Here's how the part is built. I have some questions about the finished solid (model axes, mm). A direction names the side the tool comes from. Give positions to 0.01 mm unless a question says otherwise; leave off trailing zeros. Write each loop counter-clockwise with the first axis right and the second up, starting at its lowest first coordinate (ties: lowest second). Pieces come first, ordered by that corner, then holes. Notation, with made-up numbers: (57.5, 82) -> (72.5, 82) arc R22 cw to (72.5, 120) -> close; hole circle Ø10 at (16.5, 12). An arc over 180 degrees is marked (long way). Return JSON: item names as keys, results as strings.
from build123d import *

# Parameters (mm, degrees)
BOSS_EXTRUDE5_DEPTH = 19
BOSS_EXTRUDE6_DEPTH = 8
BOSS_EXTRUDE7_DEPTH = 6.325904881
SKETCH11_R          = 1.75
CUT_MOTOR_DEPTH     = 19
SKETCH12_R          = 1.5
CUT_EXTRUDE7_DEPTH  = 46.325937613
SKETCH13_R          = 2.25
CUT_EXTRUDE8_DEPTH  = 46.216453805
SKETCH14_R          = 5.5
CUT_EXTRUDE9_DEPTH  = 4
SKETCH16_R          = 11.5
CUT_MOTOR_L_DEPTH   = 2.5
CUT_MOTOR_R_START   = -2.5
SKETCH15_R          = 11.5
CUT_MOTOR_R_DEPTH   = 2.5
SKETCH19_R          = 3.25
CUT_EXTRUDE10_DEPTH = 8
SKETCH20_R          = 2.75
CUT_EXTRUDE11_DEPTH = 62.878766896
CUT_EXTRUDE12_DEPTH = 56.924303306
FILLET1_R           = 2
FILLET2_R           = 1.5
FILLET3_R           = 1.5
SKETCH24_R          = 1.75
CUT_EXTRUDE14_DEPTH = 6
CUT_EXTRUDE15_DEPTH = 2.5


with BuildPart() as part:
    # Sketch10 → Boss-Extrude5 (new, symmetric)
    with BuildSketch(Plane(origin=(0, 0, 0), x_dir=(0, 0, -1), z_dir=(1, 0, 0))):
        with BuildLine():
            Line((-27.445904881, 9.607875665), (-20.588029216, 9.607875665))
            Line((-20.588029216, 9.607875665), (-17.838029216, 6.857875665))
            Line((-17.838029216, 6.857875665), (-17.838029216, 0))
            Line((-17.838029216, 0), (0.18, 0))
            Line((0.18, 0), (0.18, -25))
            Line((0.18, -25), (6.18, -25))
            Line((6.18, -25), (6.18, -6.648603252))
            Line((6.18, -6.648603252), (9.067622319, -3.148603252))
            Line((9.067622319, -3.148603252), (13.795773677, -3.148603252))
            ThreePointArc((13.795773677, -3.148603252), (19.7879876, -3.62453907), (22.93, 1.5))
            Line((22.93, 1.5), (22.93, 17.5))
            Line((22.93, 17.5), (-21.12, 17.5))
            Line((-21.12, 17.5), (-21.12, 25.5))
            Line((-21.12, 25.5), (-27.445904881, 25.5))
            Line((-27.445904881, 25.5), (-27.445904881, 9.607875665))
        make_face()
    extrude(amount=BOSS_EXTRUDE5_DEPTH, both=True)

    # Sketch18 → Boss-Extrude6 (add)
    with BuildSketch(Plane(origin=(0, 17.5, 0), x_dir=(1, 0, 0), z_dir=(0, 1, 0))):
        Polygon((-3.75, 22.93), (3.75, 22.93), (3.75, -21.12), (-3.75, -21.12), (-3.75, 14.93), align=None)
    extrude(amount=BOSS_EXTRUDE6_DEPTH)

    # Sketch21 → Boss-Extrude7 (add)
    with BuildSketch(Plane(origin=(0, 0, 27.445904881), x_dir=(-1, 0, 0), z_dir=(0, 0, -1))):
        with BuildLine():
            Line((8.062257748, 25.5), (-8.062257748, 25.5))
            ThreePointArc((-8.062257748, 25.5), (0, 30.5), (8.062257748, 25.5))
        make_face()
    extrude(amount=BOSS_EXTRUDE7_DEPTH)

    # Sketch11 → Cut-Motor (cut, symmetric)
    with BuildSketch(Plane(origin=(0, 0, 0), x_dir=(0, 0, -1), z_dir=(1, 0, 0))):
        with Locations((-15.47, 11.35)):
            Circle(SKETCH11_R)
        with Locations((15.53, 11.35)):
            Circle(SKETCH11_R)
        with Locations((17.18, 1.5)):
            Circle(SKETCH11_R)
    extrude(amount=CUT_MOTOR_DEPTH, both=True, mode=Mode.SUBTRACT)

    # Sketch12 → Cut-Extrude7 (cut, through all)
    with BuildSketch(Plane.XY.offset(-0.18)):
        with Locations((0, -20)):
            Circle(SKETCH12_R)
        with Locations((4.5, -10)):
            Circle(SKETCH12_R)
        with Locations((-4.5, -10)):
            Circle(SKETCH12_R)
    extrude(amount=-CUT_EXTRUDE7_DEPTH, mode=Mode.SUBTRACT)

    # Sketch13 → Cut-Extrude8 (cut, through all)
    with BuildSketch(Plane.XZ):
        with Locations(Location((-9, 5.82, 0), (0, 0, 270))):
            Circle(SKETCH13_R)
        with Locations(Location((9, 5.82, 0), (0, 0, 270))):
            Circle(SKETCH13_R)
    extrude(amount=-CUT_EXTRUDE8_DEPTH, mode=Mode.SUBTRACT)

    # Sketch14 → Cut-Extrude9 (cut)
    with BuildSketch(Plane.XZ):
        with Locations(Location((9, 5.82, 0), (0, 0, 270))):
            Circle(SKETCH14_R)
        with Locations(Location((-9, 5.82, 0), (0, 0, 270))):
            Circle(SKETCH14_R)
    extrude(amount=-CUT_EXTRUDE9_DEPTH, mode=Mode.SUBTRACT)

    # Sketch16 → Cut-Motor-L (cut)
    with BuildSketch(Plane.ZY.offset(19)):
        with Locations((-0.03, 26.85)):
            Circle(SKETCH16_R)
    extrude(amount=-CUT_MOTOR_L_DEPTH, mode=Mode.SUBTRACT)

    # Sketch15 → Cut-Motor-R (cut)
    with BuildSketch(Plane(origin=(19, 0, 0), x_dir=(0, 0, -1), z_dir=(1, 0, 0)).offset(CUT_MOTOR_R_START)):
        with Locations((0.03, 26.85)):
            Circle(SKETCH15_R)
    extrude(amount=CUT_MOTOR_R_DEPTH, mode=Mode.SUBTRACT)

    # Sketch19 → Cut-Extrude10 (cut)
    with BuildSketch(Plane(origin=(3.75, 0, 0), x_dir=(0, 0, -1), z_dir=(1, 0, 0))):
        with Locations((0.03, 26.85)):
            Circle(SKETCH19_R)
    extrude(amount=-CUT_EXTRUDE10_DEPTH, mode=Mode.SUBTRACT)

    # Sketch20 → Cut-Extrude11 (cut, through all)
    with BuildSketch(Plane.XY.offset(-22.93)):
        with Locations((0, 21.5)):
            Circle(SKETCH20_R)
    extrude(amount=CUT_EXTRUDE11_DEPTH, mode=Mode.SUBTRACT)

    # Sketch22 → Cut-Extrude12 (cut, through all)
    with BuildSketch(Plane(origin=(19, 0, 0), x_dir=(0, 0, -1), z_dir=(1, 0, 0))):
        with BuildLine():
            Line((-0.188639117, 6.801063089), (8.411360883, 2.907650311))
            ThreePointArc((8.411360883, 2.907650311), (9.843031772, 3.013589679), (10.53, 4.274136916))
            Line((10.53, 4.274136916), (10.53, 11))
            ThreePointArc((10.53, 11), (10.090660172, 12.060660172), (9.03, 12.5))
            Line((9.03, 12.5), (0.43, 12.5))
            ThreePointArc((0.43, 12.5), (-0.630660172, 12.060660172), (-1.07, 11))
            Line((-1.07, 11), (-1.07, 8.167549694))
            ThreePointArc((-1.07, 8.167549694), (-0.830547238, 7.354517922), (-0.188639117, 6.801063089))
        make_face()
    extrude(amount=-CUT_EXTRUDE12_DEPTH, mode=Mode.SUBTRACT)

    # Fillet1
    fillet1_edges = [part.edges().sort_by_distance(p)[0] for p in [
        (11.375, 17.5, 21.12),
        (-11.375, 17.5, 21.12),
    ]]
    fillet(fillet1_edges, radius=FILLET1_R)

    # Fillet2
    fillet2_edges = [part.edges().sort_by_distance(p)[0] for p in [
        (0, 30.5, 21.12),
        (0, 30.5, 27.445904881),
    ]]
    fillet(fillet2_edges, radius=FILLET2_R)

    # Fillet3
    fillet3_edges = [part.edges().sort_by_distance(p)[0] for p in [
        (3.75, 25.5, -12.95817455),
        (-3.75, 25.5, 12.02317455),
        (-3.75, 25.5, -12.95817455),
        (3.75, 25.5, 12.02317455),
    ]]
    fillet(fillet3_edges, radius=FILLET3_R)

    # Sketch24 → Cut-Extrude14 (cut)
    with BuildSketch(Plane.XZ.offset(-9.607875665)):
        with Locations(Location((-12.5, 22.445904881, 0), (0, 0, 270))):
            Circle(SKETCH24_R)
        with Locations(Location((12.5, 22.445904881, 0), (0, 0, 270))):
            Circle(SKETCH24_R)
    extrude(amount=-CUT_EXTRUDE14_DEPTH, mode=Mode.SUBTRACT)

    # Sketch25 → Cut-Extrude15 (cut)
    with BuildSketch(Plane.XZ.offset(-15.607875665)):
        Polygon((-15.667914761, 27.445904881), (-9.332085239, 27.445904881), (-9.332085239, 20.616908441), (-12.5, 18.787912001), (-15.667914761, 20.616908441), align=None)
        Polygon((9.332085239, 27.445904881), (15.667914761, 27.445904881), (15.667914761, 20.616908441), (12.5, 18.787912001), (9.332085239, 20.616908441), align=None)
    extrude(amount=CUT_EXTRUDE15_DEPTH, mode=Mode.SUBTRACT)


solid = part.part
1. If I drill on line 1 (Y direction, x = -10, z = 21.5); line 2 (Y direction, x = 10, z = 15.5); line 3 (X direction, y = 21.5, z = 10), over which ranges is the centre line in solid material (lowest first)? Write a range as [from, to].
Taken from the geometry:
{"line 1": "y = [9.61, 13.11], [15.61, 25.5]", "line 2": "y = [0, 9.6], [13.1, 17.5]", "line 3": "x = [-3.75, -2.75], [2.75, 3.75]"}
2. Suppose I cut it at C-C, the plane y = 14.5. List the corners of the cut face in (x, z) for me, and give its area (3 significant figures).
Taken from the geometry:
{"outline": "(-19, -22.93) -> (19, -22.93) -> (19, 27.45) -> (15.67, 27.45) -> (15.67, 20.62) -> (12.5, 18.79) -> (9.33, 20.62) -> (9.33, 27.45) -> (-9.33, 27.45) -> (-9.33, 20.62) -> (-12.5, 18.79) -> (-15.67, 20.62) -> (-15.67, 27.45) -> (-19, 27.45) -> close; hole circle Ø4.5 at (-9, 5.82); hole circle Ø4.5 at (9, 5.82)", "area": "1,780 mm²"}
3. Suppose I cut it at A-A, the plane y = -10. List the corners of the cut face in (x, z) for me, and give its area (3 significant figures).
Taken from the geometry:
{"outline": "(-19, -6.18) -> (-6, -6.18) -> (-6, -0.18) -> (-19, -0.18) -> close; (-3, -6.18) -> (3, -6.18) -> (3, -0.18) -> (-3, -0.18) -> close; (6, -6.18) -> (19, -6.18) -> (19, -0.18) -> (6, -0.18) -> close", "area": "192 mm²"}
4. Suppose I cut it at B-B, the plane z = 5.82. Count the separate pieces of the cut face and the enclosed holes in it, and give its area (3 significant figures).
Taken from the geometry:
{"separate pieces": "3", "enclosed holes": "1", "area": "488 mm²"}
5. Which directions (+Z, -Z, +X, -X, +Y, -Y) give clear straight access to the entire face, cutting with the end or side of a thin tool? Please do faces 1 (the face through (0.266, 3.002, -9.825)), 2 (the face through (0.266, -4.923, -7.604)), 3 (the face through (-12, 13.108, 25)), 4 (the face through (16.5, 17, 0)), 5 (the face through (3.3, 25.07, -12.11)).
Taken from the geometry:
{"face 1": "+X, -X", "face 2": "+X, -X, -Y", "face 3": "+Z", "face 4": "+X, +Y", "face 5": "-Z, +X, +Y"}
6. For pin 1 Ø1.9 at (x, z) = (13.5, 21.5) entering from -Y; pin 2 Ø5.5 at (x, z) = (11, 4) entering from -Y; pin 3 Ø4 at (x, z) = (-13, -14) entering from -Y; pin 4 Ø1.8 at (x, y) = (0, -20) entering from -Z, each with a flat end and sliding along its axis, tell me the tip position at first contact or that it passes through.
Taken from the geometry:
{"pin 1": "stops at y = 9.57", "pin 2": "stops at y = 4", "pin 3": "stops at y = -4.13", "pin 4": "passes through"}
7. If we mould it in two halves opening along Z, with no side actions, what happens to faces 6 (the face through (0.27, 4.88, -4.05)), 7 (the face through (0, 25.5, 12)), 8 (the face through (10.94, 14.38, 19.69))? For each: released by +Z, released by -Z, zero draft, split by the parting line, or undercut.
Taken from the geometry:
{"face 6": "undercut", "face 7": "zero draft", "face 8": "released by +Z"}
